Check sheet for the modelled part. Datum: model origin and axes. Units: mm. A direction names the side the tool comes from. Coordinates: 2 decimals unless noted, no trailing zeros. Loops run counter-clockwise (first coordinate to the right, second up) from the corner with the lowest first, then second, coordinate; pieces in that order, holes last.
```python
from build123d import *

# Parameters (mm, degrees)
BOSS_EXTRUDE1_DEPTH = 10
SKETCH2_R           = 2.5
CUT_EXTRUDE1_DEPTH  = 27.882385658
CUT_EXTRUDE2_REACH  = 26.835
SKETCH3_R           = 2
FILLET1_R           = 5
FILLET2_R           = 3
FILLET3_R           = 0.5


with BuildPart() as part:
    # Sketch1 → Boss-Extrude1 (new body)
    with BuildSketch(Plane.XY):
        Polygon((13, 0), (16, 0), (16, -19.1484375), (0, -19.1484375), (0, 0), (3, 0), (3, -16.1484375), (13, -16.1484375), align=None)
    extrude(amount=BOSS_EXTRUDE1_DEPTH)

    # Sketch2 → Cut-Extrude1 (cut, through all)
    with BuildSketch(Plane.ZY):
        with Locations((5, -5)):
            Circle(SKETCH2_R)
    extrude(amount=-CUT_EXTRUDE1_DEPTH, mode=Mode.SUBTRACT)

    # Sketch3 → Cut-Extrude2 (cut, up to next)
    with BuildSketch(Plane(origin=(0, -16.1484375, 0), x_dir=(1, 0, 0), z_dir=(0, 1, 0)), mode=Mode.PRIVATE) as cut_extrude2_sk1:
        with Locations(Location((8, -5, 0), (0, 0, 270))):
            Circle(SKETCH3_R)
    cut_extrude2_tool1 = extrude(cut_extrude2_sk1.sketch, amount=-CUT_EXTRUDE2_REACH, mode=Mode.PRIVATE) & part.part
    add(cut_extrude2_tool1.solids().sort_by_distance((8, -16.148438, 5))[0], mode=Mode.SUBTRACT)

    # Fillet1
    fillet1_edges = [part.edges().sort_by_distance(p)[0] for p in [
        (14.5, 0, 10),
        (14.5, 0, 0),
        (1.5, 0, 0),
        (1.5, 0, 10),
    ]]
    fillet(fillet1_edges, radius=FILLET1_R - 0.0001)  # a hair under: the kernel refuses the full size

    # Fillet2
    fillet2_edges = [part.edges().sort_by_distance(p)[0] for p in [
        (16, -19.1484375, 5),
        (0, -19.1484375, 5),
    ]]
    fillet(fillet2_edges, radius=FILLET2_R)

    # Fillet3
    fillet3_edges = [part.edges().sort_by_distance(p)[0] for p in [
        (3, -16.1484375, 5),
        (13, -16.1484375, 5),
    ]]
    fillet(fillet3_edges, radius=FILLET3_R)


solid = part.part
```
1) Scan lines: line 1 (X direction, y = -14.5, z = 4.75); line 2 (Y direction, x = 5.5, z = 6.5); line 3 (Y direction, x = 2.2, z = 5). Record each from-to range of solid material in increasing order.
Answer sheet:
line 1: x = 0 to 3, 13 to 16
line 2: y = -19.15 to -16.15
line 3: y = -19.04 to -7.5, -2.5 to 0
2) Section check C-C on y = -3. Enter the section's corners in (x, z), plus the area to 3 significant figures.
Answer sheet:
outline: (0, 0.42) - (3, 0.42) - (3, 3.5) - (0, 3.5) - close; (0, 6.5) - (3, 6.5) - (3, 9.58) - (0, 9.58) - close; (13, 0.42) - (16, 0.42) - (16, 3.5) - (13, 3.5) - close; (13, 6.5) - (16, 6.5) - (16, 9.58) - (13, 9.58) - close
area: 37.0 mm2
3) Mould release check, pull along Z, two halves, no side actions. Record for faces 3 (the flat face through (7.9, -16.148, 2.7)), 4 (the cylindrical face through (14.479, -4.249, 7.385)), 5 (the cylindrical face through (9.352, -17.627, 3.526)), 6 (the cylindrical face through (2, -2, 9)): +Z half, -Z half, draft (parallel to the pull), parting line (faces both ways), or undercut.
Answer sheet:
face 3: draft
face 4: undercut
face 5: undercut
face 6: +Z half
4) Set-up check for faces 1 (the cylindrical face through (1.479, -4.249, 7.385)), 2 (the flat face through (3, -9, 5)): record each of +Z, -Z, +X, -X, +Y, -Y from which the full face is reachable in a straight line by a thin tool's end or side.
Answer sheet:
face 1: +X, -X
face 2: +Z, -Z, +Y
5) Section check A-A on y = -9.25. Enter the section's corners in (x, z).
Answer sheet:
outline: (0, 0) - (3, 0) - (3, 10) - (0, 10) - close; (13, 0) - (16, 0) - (16, 10) - (13, 10) - close
6) Depth check by flat-ended pin: pin 1 (4 mm diameter, centred on x = 14, z = 8.5, fed in from +Y); pin 2 (4.5 mm diameter, centred on x = 9.5, z = 6, fed in from +Y). Enter the tip coordinate at first touch or a pass-through.
Answer sheet:
pin 1: stops at y = -0.23
pin 2: stops at y = -16.15
7) Section check B-B on x = 8. Enter the section's corners in (y, z).
Answer sheet:
outline: (-19.15, 0) - (-16.15, 0) - (-16.15, 3) - (-19.15, 3) - close; (-19.15, 7) - (-16.15, 7) - (-16.15, 10) - (-19.15, 10) - close
